from build123d import *

# Parameters (mm, degrees)
ESQUISSE1_R        = 1.6
BOSS_EXTRU_1_DEPTH = 5
CONG_1_R           = 1


with BuildPart() as part:
    # Esquisse1 → Boss.-Extru.1 (new body)
    with BuildSketch(Plane(origin=(0, 0, 0), x_dir=(-1, 0, 0), z_dir=(0, 0, -1))):
        with BuildLine():
            Line((-29.61, 24.250000923), (-29.61, 10))
            Line((-29.61, 10), (-18.900000032, 10))
            Line((-18.900000032, 10), (-18.866500027, 10.125000016))
            Line((-18.866500027, 10.125000016), (-18.775000016, 10.216510027))
            Line((-18.775000016, 10.216510027), (-18.65, 10.250000032))
            Line((-18.65, 10.250000032), (-18.524999984, 10.216510027))
            Line((-18.524999984, 10.216510027), (-18.433489973, 10.125000016))
            Line((-18.433489973, 10.125000016), (-18.399999968, 10))
            Line((-18.399999968, 10), (-18.433489973, 9.874995396))
            Line((-18.433489973, 9.874995396), (-18.524999984, 9.783488385))
            Line((-18.524999984, 9.783488385), (-18.65, 9.74999538))
            Line((-18.65, 9.74999538), (-18.65, 0.499994211))
            ThreePointArc((-18.65, 0.499994211), (-18.503553372, 0.146440776), (-18.149999937, -5.852e-06))
            Line((-18.149999937, -5.852e-06), (-12.150000163, -5.852e-06))
            ThreePointArc((-12.150000163, -5.852e-06), (-11.796446657, 0.146440805), (-11.65, 0.499994311))
            Line((-11.65, 0.499994311), (-11.65, 9.74999538))
            Line((-11.65, 9.74999538), (-11.775000016, 9.783488385))
            Line((-11.775000016, 9.783488385), (-11.866510027, 9.874995396))
            Line((-11.866510027, 9.874995396), (-11.900000032, 9.999995412))
            Line((-11.900000032, 9.999995412), (-11.866510027, 10.124995428))
            Line((-11.866510027, 10.124995428), (-11.775000016, 10.216505439))
            Line((-11.775000016, 10.216505439), (-11.65, 10.249995444))
            Line((-11.65, 10.249995444), (-11.524999984, 10.216505439))
            Line((-11.524999984, 10.216505439), (-11.433489973, 10.124995428))
            Line((-11.433489973, 10.124995428), (-11.399999968, 9.999995412))
            Line((-11.399999968, 9.999995412), (-0.499947825, 9.999995412))
            ThreePointArc((-0.499947825, 9.999995412), (-0.14639439, 10.14644204), (5.2238e-05, 10.499995475))
            Line((5.2238e-05, 10.499995475), (5.2238e-05, 15.499995349))
            ThreePointArc((5.2238e-05, 15.499995349), (-0.14639439, 15.853548784), (-0.499947825, 15.999995412))
            Line((-0.499947825, 15.999995412), (-7.49994871, 15.999995412))
            ThreePointArc((-7.49994871, 15.999995412), (-7.853502145, 16.14644204), (-7.999948773, 16.499995475))
            Line((-7.999948773, 16.499995475), (-7.999948773, 47.071569339))
            ThreePointArc((-7.999948773, 47.071569339), (-8.152190984, 47.836942158), (-8.585740096, 48.485793767))
            Line((-8.585740096, 48.485793767), (-11.814159255, 51.714209926))
            ThreePointArc((-11.814159255, 51.714209926), (-12.46301048, 52.147758127), (-13.228382526, 52.3))
            Line((-13.228382526, 52.3), (-29.61, 52.3))
            Line((-29.61, 52.3), (-29.61, 38.049999077))
            ThreePointArc((-29.61, 38.049999077), (-29.492842932, 37.767156996), (-29.210000822, 37.65))
            ThreePointArc((-29.210000822, 37.65), (-22.71, 31.15), (-29.210000822, 24.65))
            ThreePointArc((-29.210000822, 24.65), (-29.492842932, 24.532843004), (-29.61, 24.250000923))
        make_face()
        with Locations((-13.61, 46.65)):
            Circle(ESQUISSE1_R, mode=Mode.SUBTRACT)
        with Locations((-13.61, 15.65)):
            Circle(ESQUISSE1_R, mode=Mode.SUBTRACT)
        with BuildLine():
            Line((-22.400002831, 14.000001769), (-26.900003431, 14.000001769))
            ThreePointArc((-26.900003431, 14.000001769), (-27.326780127, 13.823225074), (-27.150003431, 14.250001769))
            Line((-27.150003431, 14.250001769), (-27.150003431, 16.250002022))
            ThreePointArc((-27.150003431, 16.250002022), (-27.326780127, 16.676778718), (-26.900003431, 16.500002022))
            Line((-26.900003431, 16.500002022), (-22.400002831, 16.500002022))
            ThreePointArc((-22.400002831, 16.500002022), (-21.973226158, 16.676778803), (-22.150002831, 16.250002085))
            Line((-22.150002831, 16.250002085), (-22.150002831, 14.250001769))
            ThreePointArc((-22.150002831, 14.250001769), (-21.973226136, 13.823225074), (-22.400002831, 14.000001769))
        make_face(mode=Mode.SUBTRACT)
    extrude(amount=-BOSS_EXTRU_1_DEPTH)

    # Congé1
    cong_1_edges = [part.edges().sort_by_distance(p)[0] for p in [
        (29.61, 10, 2.5),
        (29.61, 52.3, 2.5),
    ]]
    fillet(cong_1_edges, radius=CONG_1_R)


solid = part.part
Input: part model. Units: mm. Frame: model coordinates. A direction names the side the tool comes from. Give positions to 0.01 mm unless a question says otherwise; leave off trailing zeros. Loops run counter-clockwise (first coordinate to the right, second up) from the corner with the lowest first, then second, coordinate; pieces in that order, holes last. Notation, with made-up numbers: (58, 4.25) -> (84, 4.25) arc R24 cw to (84, 27.25) -> close; hole circle Ø3 at (81.5, 22). An arc over 180 degrees is marked (long way). Answer as a JSON object with one key per item and string values. Group by question number.
Item 1: Cut plane A-A, the plane y = 31.15. Return the cut outline in (x, z), and give its area (3 significant figures).
Item 2: Cut plane C-C, the plane y = 9. Return the cut outline in (x, z).
Item 3: Cut plane B-B, the plane z = 3.95. State how many separate pieces and enclosed holes the cut face has, and give its area (3 significant figures).
Item 4: Pin query (flat end, axial travel): P1, Ø3, axis at x = 26, z = 1, coming from the -Y side; P2, Ø1.5, axis at y = 3.5, z = 2.5, coming from the +X side; P3, Ø1.5, axis at y = 30, z = 2, coming from the -X side. Return the tip coordinate at first contact, or that it passes through.
Item 5: Pull-direction query (X, two-part tool) for faces 1 (the flat face through (22.15, 15, 2)), 2 (the flat face through (15, 0, 2)), 3 (the cylindrical face through (8.15, 47.83, 2.46)); classes: released by +X, released by -X, zero draft, split by the parting line, or undercut.
Item 6: Line query: probe 1 along X at (y, z) = (15.5, 3.65); probe 2 along Y at (x, z) = (13.61, 1.1); probe 3 along Y at (x, z) = (22.5, 3.9). Output: solid intervals per line, ascending.
Item 7: Reachability of faces 4 (the flat face through (25, 16.5, 2)), 5 (the flat face through (4, 16, 2)), 6 (the flat face through (29.61, 45, 2)), 7 (the flat face through (11.65, 5, 2)), 8 (the flat face through (18.65, 5, 2)) from +Z, -Z, +X, -X, +Y, -Y: full face, straight path, thin tool, end or side. Return the list, or none.
Checks:
{
 "1": {"outline": "(8, 0) -> (22.71, 0) -> (22.71, 5) -> (8, 5) -> close", "area": "73.6 mm²"},
 "2": {"outline": "(11.65, 0) -> (18.65, 0) -> (18.65, 5) -> (11.65, 5) -> close"},
 "3": {"separate pieces": "1", "enclosed holes": "3", "area": "921 mm²"},
 "4": {"P1": "stops at y = 10", "P2": "stops at x = 18.65", "P3": "stops at x = 8"},
 "5": {"face 1": "undercut", "face 2": "zero draft", "face 3": "released by -X"},
 "6": {"probe 1": "x = 0 to 12.02, 15.2 to 22.15, 27.15 to 29.61", "probe 2": "y = 0 to 14.05, 17.25 to 45.05, 48.25 to 52.3", "probe 3": "y = 10 to 14, 16.5 to 52.3"},
 "7": {"face 4": "+Z, -Z", "face 5": "+Z, -Z, -X, +Y", "face 6": "+Z, -Z, +X, +Y, -Y", "face 7": "+Z, -Z, -X, -Y", "face 8": "+Z, -Z, +X, -Y"}
}
